from build123d import *

# Parameters (mm, degrees)
EXTRUDE_1_DEPTH          = 5
CUT_EXTRUDE_2_DEPTH      = 115.952164093
CUT_EXTRUDE_2_DEPTH_BACK = 115.952164093
SKETCH_3_OUTSIDE_W       = 97.176
SKETCH_3_OUTSIDE_H       = 161.176
SKETCH_3_OUTSIDE_R       = 7.5
SKETCH_4_R               = 7.5
CUT_EXTRUDE_3_DEPTH      = 115.952164093
SKETCH_5_R               = 1.5
CUT_EXTRUDE_4_DEPTH      = 5


with BuildPart() as part:
    # 草图1 → 凸台-拉伸1 (new body)
    with BuildSketch(Plane.XY):
        with BuildLine():
            Line((-20, 0), (-20, -50))
            Line((-20, -50), (-20, -74.091630608))
            add(Edge.make_bspline(
                [(-2.03e-07, -70), (-11.13946442, -70.000000042), (-20, -74.091630608)],
                knots=[4.712388987, 4.712388987, 4.712388987, 5.363487565, 5.363487565, 5.363487565], degree=2, weights=[1, 0.947475191, 1]))
            add(Edge.make_bspline(
                [(20, -74.091630608), (11.13946424, -69.999999958), (-2.03e-07, -70)],
                knots=[4.061290395, 4.061290395, 4.061290395, 4.712388987, 4.712388987, 4.712388987], degree=2, weights=[1, 0.947475189, 1]))
            Line((20, -74.091630608), (20, -50))
            Line((20, -50), (20, 0))
            ThreePointArc((20, 0), (0, -20), (-20, 0))
        make_face()
        with BuildLine():
            Line((-20, -74.091630608), (-20, -50))
            Line((-20, -50), (-32.310858712, -85.934042004))
            add(Edge.make_bspline(
                [(-20, -74.091630608), (-29.804870228, -78.619337355), (-32.310858712, -85.934042004)],
                knots=[5.363487565, 5.363487565, 5.363487565, 6.078460318, 6.078460318, 6.078460318], degree=2, weights=[1, 0.936779351, 1]))
        make_face()
        with BuildLine():
            add(Edge.make_bspline(
                [(-20, -74.091630608), (-29.804870228, -78.619337355), (-32.310858712, -85.934042004)],
                knots=[5.363487565, 5.363487565, 5.363487565, 6.078460318, 6.078460318, 6.078460318], degree=2, weights=[1, 0.936779351, 1]))
            add(Edge.make_bspline(
                [(-32.310858712, -85.934042004), (-33, -87.945569596), (-33, -90)],
                knots=[6.078460318, 6.078460318, 6.078460318, 6.283185307, 6.283185307, 6.283185307], degree=2, weights=[1, 0.994765533, 1]))
            add(Edge.make_bspline(
                [(-33, -90), (-33, -109.999999875), (-2.06e-07, -110)],
                knots=[0, 0, 0, 1.570796321, 1.570796321, 1.570796321], degree=2, weights=[1, 0.707106783, 1]))
            ThreePointArc((-2.06e-07, -110), (-14.142135697, -104.142135551), (-20, -90))
            Line((-20, -90), (-20, -74.091630608))
        make_face()
        with BuildLine():
            add(Edge.make_bspline(
                [(-2.03e-07, -70), (-11.13946442, -70.000000042), (-20, -74.091630608)],
                knots=[4.712388987, 4.712388987, 4.712388987, 5.363487565, 5.363487565, 5.363487565], degree=2, weights=[1, 0.947475191, 1]))
            Line((-20, -74.091630608), (-20, -90))
            ThreePointArc((-20, -90), (-14.142135696, -75.857864448), (-2.03e-07, -70))
        make_face()
        with BuildLine():
            add(Edge.make_bspline(
                [(-20, -74.091630608), (-29.804870228, -78.619337355), (-32.310858712, -85.934042004)],
                knots=[5.363487565, 5.363487565, 5.363487565, 6.078460318, 6.078460318, 6.078460318], degree=2, weights=[1, 0.936779351, 1]))
            add(Edge.make_bspline(
                [(-32.310858712, -85.934042004), (-33, -87.945569596), (-33, -90)],
                knots=[6.078460318, 6.078460318, 6.078460318, 6.283185307, 6.283185307, 6.283185307], degree=2, weights=[1, 0.994765533, 1]))
            add(Edge.make_bspline(
                [(-33, -90), (-33, -109.999999875), (-2.06e-07, -110)],
                knots=[0, 0, 0, 1.570796321, 1.570796321, 1.570796321], degree=2, weights=[1, 0.707106783, 1]))
            ThreePointArc((-2.06e-07, -110), (-14.142135697, -104.142135551), (-20, -90))
            Line((-20, -90), (-20, -74.091630608))
        make_face()
        with BuildLine():
            add(Edge.make_bspline(
                [(-2.03e-07, -70), (-11.13946442, -70.000000042), (-20, -74.091630608)],
                knots=[4.712388987, 4.712388987, 4.712388987, 5.363487565, 5.363487565, 5.363487565], degree=2, weights=[1, 0.947475191, 1]))
            Line((-20, -74.091630608), (-20, -90))
            ThreePointArc((-20, -90), (-14.142135696, -75.857864448), (-2.03e-07, -70))
        make_face()
        with BuildLine():
            add(Edge.make_bspline(
                [(20, -74.091630608), (11.13946424, -69.999999958), (-2.03e-07, -70)],
                knots=[4.061290395, 4.061290395, 4.061290395, 4.712388987, 4.712388987, 4.712388987], degree=2, weights=[1, 0.947475189, 1]))
            ThreePointArc((-2.03e-07, -70), (14.142135552, -75.857864304), (20, -90))
            Line((20, -90), (20, -74.091630608))
        make_face()
        with BuildLine():
            ThreePointArc((20, -90), (14.142135551, -104.142135697), (-2.06e-07, -110))
            add(Edge.make_bspline(
                [(-2.06e-07, -110), (40.555759481, -110.000000153), (32.310858712, -85.934042004)],
                knots=[1.570796321, 1.570796321, 1.570796321, 3.346317643, 3.346317643, 3.346317643], degree=2, weights=[1, 0.631150574, 1]))
            add(Edge.make_bspline(
                [(32.310858712, -85.934042004), (29.804870228, -78.619337355), (20, -74.091630608)],
                knots=[3.346317643, 3.346317643, 3.346317643, 4.061290395, 4.061290395, 4.061290395], degree=2, weights=[1, 0.936779351, 1]))
            Line((20, -74.091630608), (20, -90))
        make_face()
        with BuildLine():
            Line((32.310858712, -85.934042004), (20, -50))
            Line((20, -50), (20, -74.091630608))
            add(Edge.make_bspline(
                [(32.310858712, -85.934042004), (29.804870228, -78.619337355), (20, -74.091630608)],
                knots=[3.346317643, 3.346317643, 3.346317643, 4.061290395, 4.061290395, 4.061290395], degree=2, weights=[1, 0.936779351, 1]))
        make_face()
        with BuildLine():
            add(Edge.make_bspline(
                [(20, -74.091630608), (11.13946424, -69.999999958), (-2.03e-07, -70)],
                knots=[4.061290395, 4.061290395, 4.061290395, 4.712388987, 4.712388987, 4.712388987], degree=2, weights=[1, 0.947475189, 1]))
            ThreePointArc((-2.03e-07, -70), (14.142135552, -75.857864304), (20, -90))
            Line((20, -90), (20, -74.091630608))
        make_face()
        with BuildLine():
            ThreePointArc((20, -90), (14.142135551, -104.142135697), (-2.06e-07, -110))
            add(Edge.make_bspline(
                [(-2.06e-07, -110), (40.555759481, -110.000000153), (32.310858712, -85.934042004)],
                knots=[1.570796321, 1.570796321, 1.570796321, 3.346317643, 3.346317643, 3.346317643], degree=2, weights=[1, 0.631150574, 1]))
            add(Edge.make_bspline(
                [(32.310858712, -85.934042004), (29.804870228, -78.619337355), (20, -74.091630608)],
                knots=[3.346317643, 3.346317643, 3.346317643, 4.061290395, 4.061290395, 4.061290395], degree=2, weights=[1, 0.936779351, 1]))
            Line((20, -74.091630608), (20, -90))
        make_face()
        with BuildLine():
            ThreePointArc((20, 0), (0, 20), (-20, 0))
            Line((-20, 0), (20, 0))
        make_face()
        with BuildLine():
            Line((20, 0), (-20, 0))
            ThreePointArc((-20, 0), (0, -20), (20, 0))
        make_face()
        with BuildLine():
            ThreePointArc((20, 0), (0, 20), (-20, 0))
            Line((-20, 0), (20, 0))
        make_face()
        with BuildLine():
            Line((20, 0), (-20, 0))
            ThreePointArc((-20, 0), (0, -20), (20, 0))
        make_face()
        with BuildLine():
            ThreePointArc((-2.03e-07, -70), (-14.142135696, -75.857864448), (-20, -90))
            Line((-20, -90), (20, -90))
            ThreePointArc((20, -90), (14.142135552, -75.857864304), (-2.03e-07, -70))
        make_face()
        with BuildLine():
            Line((20, -90), (-20, -90))
            ThreePointArc((-20, -90), (-14.142135697, -104.142135551), (-2.06e-07, -110))
            ThreePointArc((-2.06e-07, -110), (14.142135551, -104.142135697), (20, -90))
        make_face()
        with BuildLine():
            ThreePointArc((-2.03e-07, -70), (-14.142135696, -75.857864448), (-20, -90))
            Line((-20, -90), (20, -90))
            ThreePointArc((20, -90), (14.142135552, -75.857864304), (-2.03e-07, -70))
        make_face()
        with BuildLine():
            Line((20, -90), (-20, -90))
            ThreePointArc((-20, -90), (-14.142135697, -104.142135551), (-2.06e-07, -110))
            ThreePointArc((-2.06e-07, -110), (14.142135551, -104.142135697), (20, -90))
        make_face()
    extrude(amount=EXTRUDE_1_DEPTH)

    # 草图3 outside → 切除-拉伸2 (cut, two sides: drawn at the far end of the back side and taken through both)
    # profile 1 of 2: a face of its own
    with BuildSketch(Plane.XY.offset(5).offset(-CUT_EXTRUDE_2_DEPTH_BACK)):
        with Locations((0, -45)):
            Rectangle(SKETCH_3_OUTSIDE_W, SKETCH_3_OUTSIDE_H)
        with BuildLine():
            Line((32.310858712, -85.934042004), (20, -50))
            Line((20, -50), (20, 0))
            ThreePointArc((20, 0), (0, 20), (-20, 0))
            Line((-20, 0), (-20, -50))
            Line((-20, -50), (-32.310858712, -85.934042004))
            add(Edge.make_bspline(
                [(-32.310858712, -85.934042004), (-40.555759429, -110), (0, -110), (40.555759429, -110), (32.310858712, -85.934042004)],
                knots=[6.078460318, 6.078460318, 6.078460318, 7.853981634, 7.853981634, 9.62950295, 9.62950295, 9.62950295], degree=2, weights=[1, 0.631150576, 1, 0.631150576, 1]))
        make_face(mode=Mode.SUBTRACT)
    # profile 2 of 2: a face of its own
    with BuildSketch(Plane.XY.offset(5).offset(-CUT_EXTRUDE_2_DEPTH_BACK)):
        with Locations((0, -90)):
            Circle(SKETCH_3_OUTSIDE_R)
    extrude(amount=CUT_EXTRUDE_2_DEPTH + CUT_EXTRUDE_2_DEPTH_BACK, mode=Mode.SUBTRACT)

    # 草图4 → 切除-拉伸3 (cut, through all)
    with BuildSketch(Plane.XY.offset(5)):
        Circle(SKETCH_4_R)
    extrude(amount=-CUT_EXTRUDE_3_DEPTH, mode=Mode.SUBTRACT)

    # 草图5 → 切除-拉伸4 (cut)
    with BuildSketch(Plane.XY.offset(5)):
        with Locations((28, -90)):
            Circle(SKETCH_5_R)
        with Locations((14, 0)):
            Circle(SKETCH_5_R)
        with Locations((10, -35)):
            Circle(SKETCH_5_R)
        with Locations((10, -65)):
            Circle(SKETCH_5_R)
        with Locations((-14, 0)):
            Circle(SKETCH_5_R)
        with Locations((-10, -35)):
            Circle(SKETCH_5_R)
        with Locations((-10, -65)):
            Circle(SKETCH_5_R)
        with Locations((-28, -90)):
            Circle(SKETCH_5_R)
    extrude(amount=-CUT_EXTRUDE_4_DEPTH, mode=Mode.SUBTRACT)


solid = part.part
Work out the finished part from the listing and answer in its coordinate system (mm). A direction names the side the tool comes from. Give positions to 0.01 mm unless a question says otherwise; leave off trailing zeros. Loops run counter-clockwise (first coordinate to the right, second up) from the corner with the lowest first, then second, coordinate; pieces in that order, holes last. Notation, with made-up numbers: (75.25, 80.25) -> (114.25, 80.25) arc R28 cw to (114.25, 105.25) -> close; hole circle Ø2 at (83.5, -18). An arc over 180 degrees is marked (long way). Use a Markdown table: item, result. Add a question column.
1) The part is cut by section A-A, the plane y = -65. Determine the outline of the cut face in (x, z), plus the area to 3 significant figures.
2) The part is cut by section B-B, the plane y = -90. Count the separate pieces of the cut face and the enclosed holes in it, plus the area to 3 significant figures.
3) Consider line 1 along X through (y, z) = (-90, 3.7); line 2 along Y through (x, z) = (-1.5, 3.65); line 3 along Y through (x, z) = (-3.5, 0.35). Determine where each line is inside the solid, lowest interval first.
4) For a pull along Y with two mould halves and no side action, classify faces 3 (the flat face through (-26.07, -67.72, 2.46)), 4 (the flat face through (-20, -25, 2)), 5 (the cylindrical face through (27.805, -88.513, 2.535)) as +Y half, -Y half, draft (parallel to the pull), parting line (faces both ways), or undercut.
5) Which of the six approach directions +Z, -Z, +X, -X, +Y, -Y give full straight-line access (tool end or side, diameter ignored) to faces 1 (the flat face through (20, -25, 2)), 2 (the cylindrical face through (9.675, -36.464, 2.535))?
6) Each of these flat-tipped pins is pushed along its axis until it touches: P1, Ø1.5, axis at x = -3, z = 4, coming from the -Y side; P2, Ø2.5, axis at x = -14, y = 0, coming from the -Z side; P3, Ø1, axis at y = 3.5, z = 1.5, coming from the -X side; P4, Ø2.5, axis at y = -18, z = 2, coming from the -X side. Where does it stop, or does it pass through?
Reported:
| question | item | result |
|---|---|---|
| 1 | outline | (-25.14, 0) -> (-11.5, 0) -> (-11.5, 5) -> (-25.14, 5) -> close; (-8.5, 0) -> (8.5, 0) -> (8.5, 5) -> (-8.5, 5) -> close; (11.5, 0) -> (25.14, 0) -> (25.14, 5) -> (11.5, 5) -> close |
| 1 | area | 221 mm^2 |
| 2 | separate pieces | 4 |
| 2 | enclosed holes | 0 |
| 2 | area | 225 mm^2 |
| 3 | line 1 | x = -33 to -29.5, -26.5 to -7.5, 7.5 to 26.5, 29.5 to 33 |
| 3 | line 2 | y = -109.98 to -97.35, -82.65 to -7.35, 7.35 to 19.94 |
| 3 | line 3 | y = -109.89 to -96.63, -83.37 to -6.63, 6.63 to 19.69 |
| 4 | face 3 | +Y half |
| 4 | face 4 | draft |
| 4 | face 5 | undercut |
| 5 | face 1 | +Z, -Z, +X, +Y |
| 5 | face 2 | +Z, -Z |
| 6 | P1 | stops at y = -109.95 |
| 6 | P2 | passes through |
| 6 | P3 | stops at x = -19.77 |
| 6 | P4 | stops at x = -20 |
